```python
from build123d import *

# Parameters (mm, degrees)
SKETCH_2_R = 0.9


with BuildPart() as part:
    # По траектории1: sweep along a path in Эскиз1
    with BuildLine(Plane.XY) as sweep_1_path:
        Line((-33.8, 25.3), (33.8, 25.3))
        ThreePointArc((33.8, 25.3), (34.860660172, 24.860660172), (35.3, 23.8))
        Line((35.3, 23.8), (35.3, -23.8))
        ThreePointArc((35.3, -23.8), (34.860660172, -24.860660172), (33.8, -25.3))
        Line((33.8, -25.3), (-33.8, -25.3))
        ThreePointArc((-33.8, -25.3), (-34.860660172, -24.860660172), (-35.3, -23.8))
        Line((-35.3, -23.8), (-35.3, 23.8))
        ThreePointArc((-35.3, 23.8), (-34.860660172, 24.860660172), (-33.8, 25.3))
    # Эскиз2 → По траектории1 (sweep)
    with BuildSketch(Plane(origin=(0, 0, 0), x_dir=(-1, 0, 0), z_dir=(0, -1, 0))):
        with Locations((35.3, 0)):
            Circle(SKETCH_2_R)
    sweep(path=sweep_1_path.line)


solid = part.part
```
Here's how the part is built. I have some questions about the finished solid (model axes, mm). Coordinates: 2 decimals unless noted, no trailing zeros. Order: outer loops, then holes, each group sorted by start corner. A loop starts at its lowest first (then second) coordinate and runs counter-clockwise, first axis right, second up. Notation, with made-up numbers: (36.25, 39.5) - (72.25, 39.5) arc R19 ccw to (72.25, 58.5) - close; hole circle Ø5 at (26.5, -31). An arc over 180 degrees is marked (long way). One line per question, with ' | ' between items. Start each with the question number.
1. If we section it at C-C (y = 1): Write out the boundary of the cut face in (x, z).
2. If we section it at A-A (z = -0.3): Write out the boundary of the cut face in (x, y).
3. If we section it at B-B (x = -23.5): Write out the boundary of the cut face in (y, z).
4. Please list where these lines run through material, in increasing order: line 1 along X through (y, z) = (-6, -0.05); line 2 along Y through (x, z) = (28.5, 0.1); line 3 along X through (y, z) = (17, 0.35). Write a range as [from, to].
Model answer:
1) outline: circle Ø1.8 at (-35.3, 0); circle Ø1.8 at (35.3, 0)
2) outline: (-36.15, -23.8) arc R2.35 ccw to (-33.8, -26.15) - (33.8, -26.15) arc R2.35 ccw to (36.15, -23.8) - (36.15, 23.8) arc R2.35 ccw to (33.8, 26.15) - (-33.8, 26.15) arc R2.35 ccw to (-36.15, 23.8) - close; hole (-34.45, -23.8) arc R0.65 ccw to (-33.8, -24.45) - (33.8, -24.45) arc R0.65 ccw to (34.45, -23.8) - (34.45, 23.8) arc R0.65 ccw to (33.8, 24.45) - (-33.8, 24.45) arc R0.65 ccw to (-34.45, 23.8) - close
3) outline: circle Ø1.8 at (-25.3, 0); circle Ø1.8 at (25.3, 0)
4) line 1: x = [-36.2, -34.4], [34.4, 36.2] | line 2: y = [-26.19, -24.41], [24.41, 26.19] | line 3: x = [-36.13, -34.47], [34.47, 36.13]
